CAD build for the part. Positions are in the model's coordinates, mm. Face numbers are marked on the shaded views. A direction names the side the tool comes from. Round coordinates to 2 decimals unless told otherwise and drop trailing zeros. Order: outer loops, then holes, each group sorted by start corner. A loop starts at its lowest first (then second) coordinate and runs counter-clockwise, first axis right, second up. Notation, with made-up numbers: M 71,17 L 81,17 A26 ccw 81,47 Z; hole C -4,40.5 d4. An arc over 180 degrees is marked long. Put each result on its own line as item: value.
```python
from build123d import *

# Parameters (mm, degrees)
SKETCH1_W            = 9
SKETCH1_H            = 9
BOSS_EXTRUDE1_DEPTH  = 4.5
SKETCH3_W            = 1.096908344
SKETCH3_H            = 1.096908344
BOSS_EXTRUDE3_DEPTH  = 3.5
LPATTERN1_COUNT      = 4
LPATTERN1_PITCH      = 2.54
LPATTERN1_COUNT_DIR2 = 4
LPATTERN1_PITCH_DIR2 = 2.54
SKETCH4_R            = 2.5
BOSS_EXTRUDE4_DEPTH  = 8


with BuildPart() as part:
    # Sketch1 → Boss-Extrude1 (new body)
    with BuildSketch(Plane(origin=(0, 0, 0), x_dir=(1, 0, 0), z_dir=(0, 1, 0))):
        Rectangle(SKETCH1_W, SKETCH1_H)
    extrude(amount=BOSS_EXTRUDE1_DEPTH)

    # Sketch3 → Boss-Extrude3 (add)
    with BuildSketch(Plane.XZ):
        with Locations((-3.81, 3.81)):
            Rectangle(SKETCH3_W, SKETCH3_H)
    boss_extrude3 = extrude(amount=BOSS_EXTRUDE3_DEPTH)

    # LPattern1: Boss-Extrude3 4 × 4
    with Locations(*[(i * LPATTERN1_PITCH, 0, -j * LPATTERN1_PITCH_DIR2) for i in range(LPATTERN1_COUNT) for j in range(LPATTERN1_COUNT_DIR2) if (i, j) != (0, 0)]):
        add(boss_extrude3)

    # Sketch4 → Boss-Extrude4 (add)
    with BuildSketch(Plane(origin=(0, 4.5, 0), x_dir=(1, 0, 0), z_dir=(0, 1, 0))):
        Circle(SKETCH4_R)
    extrude(amount=BOSS_EXTRUDE4_DEPTH)

    # Sketch6 → Cut-Revolve2 (revolve, cut)
    with BuildSketch(Plane(origin=(0, 0, 0), x_dir=(-0.707106781, 0, -0.707106781), z_dir=(0.707106781, 0, -0.707106781))):
        with BuildLine():
            Line((-8.778012628, -0.773952942), (-8.778012628, 5.788941631))
            Line((-8.778012628, 5.788941631), (-4.42783745, 5.788941631))
            Line((-4.42783745, 5.788941631), (-4.42783745, 4.5))
            ThreePointArc((-4.42783745, 4.5), (-7.110011532, 2.281289505), (-8.778012628, -0.773952942))
        make_face()
    revolve(axis=Axis((0, 4.5, 0), (0, -1, 0)), mode=Mode.SUBTRACT)


solid = part.part
```
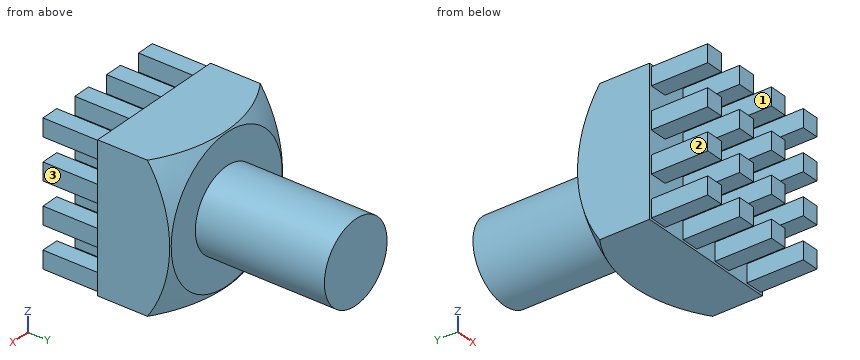
Item 1: Band-saw the part on D-D on z = 0. Give the cut face in (x, y), and give its area (3 significant figures).
Answers below:
outline: M -4.5,0 L 4.5,0 L 4.5,4.46 A9.22 ccw 4.43,4.5 L 2.5,4.5 L 2.5,12.5 L -2.5,12.5 L -2.5,4.5 L -4.43,4.5 A9.22 ccw -4.5,4.46 Z
area: 80.5 mm²
Item 2: Tool access for the marked faces 1, 2 and 3: list every direction of +Z, -Z, +X, -X, +Y, -Y with a clear straight run to the whole face (end or side of a thin tool).
Answers below:
face 1: +Z, -Z, -Y
face 2: +Z, -Z, -X, -Y
face 3: +Z, -Z, +X, -Y
Item 3: Band-saw the part on C-C on y = 10.25. Give the cut face in (x, z).
Answers below:
outline: C 0,0 d5
Item 4: Band-saw the part on B-B on x = 0. Give the cut face in (y, z), and give its area (3 significant figures).
Answers below:
outline: M 0,-4.5 L 4.46,-4.5 A9.22 ccw 4.5,-4.43 L 4.5,-2.5 L 12.5,-2.5 L 12.5,2.5 L 4.5,2.5 L 4.5,4.43 A9.22 ccw 4.46,4.5 L 0,4.5 Z
area: 80.5 mm²
Item 5: Band-saw the part on A-A on z = 3.75. Give the cut face in (x, y), and give its area (3 significant figures).
Answers below:
outline: M -4.5,0 L -4.36,0 L -4.36,-3.5 L -3.26,-3.5 L -3.26,0 L -1.82,0 L -1.82,-3.5 L -0.72,-3.5 L -0.72,0 L 0.72,0 L 0.72,-3.5 L 1.82,-3.5 L 1.82,0 L 3.26,0 L 3.26,-3.5 L 4.36,-3.5 L 4.36,0 L 4.5,0 L 4.5,3.53 A8.42 ccw 2.35,4.5 L -2.35,4.5 A8.42 ccw -4.5,3.53 Z
area: 54.0 mm²
Item 6: Pin check, flat tips, straight feed: P1, Ø0.9, axis at x = 1.5, y = -1.5, coming from the -Z side; P2, Ø3, axis at y = 10.5, z = -2.5, coming from the -X side; P3, Ø0.9, axis at y = -2, z = -1, coming from the +X side. Stop position of each tip, or through.
Answers below:
P1: z = -4.36
P2: x = -2.29
P3: x = 4.36
Item 7: Probe line 1 along X through (y, z) = (-1.5, 4); line 2 along Y through (x, z) = (1.75, 2.75). List the from-to ranges inside material, lowest first. Write a range as [from, to].
Answers below:
line 1: [-4.36, -3.26], [-1.82, -0.72], [0.72, 1.82], [3.26, 4.36]
line 2: [0, 4.5]
